```python
from build123d import *

# Parameters (mm, degrees)
F0_W     = 400
F0_H     = 900
F1_DEPTH = 200
F2_SIZE  = 50
F3_R     = 25
F4_R     = 50
F5_DEPTH = 200.001


with BuildPart() as f1:
    # F0 (on Front) → F1 (new body)
    with BuildSketch(Plane.XZ):
        with Locations((0, -35.980602)):
            Rectangle(F0_W, F0_H)
    extrude(amount=F1_DEPTH)

    # F2
    f2_edges = [f1.edges().sort_by_distance(p)[0] for p in [
        (-200, -100, 414.019398),
        (200, -100, 414.019398),
    ]]
    chamfer(f2_edges, length=F2_SIZE)

    # F3
    f3_edges = [f1.edges().sort_by_distance(p)[0] for p in [
        (-200, -100, -485.980602),
        (200, -100, -485.980602),
    ]]
    fillet(f3_edges, radius=F3_R)

    # F4 (on face) → F5 (cut, through all)
    with BuildSketch(Plane.XZ.offset(200)):
        Circle(F4_R)
    extrude(amount=-F5_DEPTH, mode=Mode.SUBTRACT)


solid = f1.part
```
Input: part model. Units: mm. Frame: model coordinates. Coordinates: 2 decimals unless noted, no trailing zeros. Write each loop counter-clockwise with the first axis right and the second up, starting at its lowest first coordinate (ties: lowest second). Pieces come first, ordered by that corner, then holes. Notation, with made-up numbers: M 67,42.5 L 72,42.5 A18 cw 72,58.5 Z; hole C 60.5,77 d7. An arc over 180 degrees is marked long. Use one line per item in the form item = value.
Q1. Section A-A (z = 0). Return loops of the section in (x, y), plus the area to 3 significant figures.
Answer below:
outline = M -200,-200 L -50,-200 L -50,0 L -200,0 Z; M 50,-200 L 200,-200 L 200,0 L 50,0 Z
area = 60,000 mm²
Q2. Section B-B (x = 0). Return loops of the section in (y, z).
Answer below:
outline = M -200,-485.98 L 0,-485.98 L 0,-50 L -200,-50 Z; M -200,50 L 0,50 L 0,414.02 L -200,414.02 Z
Q3. Material intervals for probe 1 along Z at (x, y) = (0, -64); probe 2 along Z at (x, y) = (13, -135); probe 3 along X at (y, z) = (-44.5, -9), sorted ascending. Write a range as from..to.
Answer below:
probe_1 = -485.98..-50, 50..414.02
probe_2 = -485.98..-48.28, 48.28..414.02
probe_3 = -200..-49.18, 49.18..200
Q4. Section C-C (y = -76.5). Return loops of the section in (x, z).
Answer below:
outline = M -200,-460.98 A25 ccw -175,-485.98 L 175,-485.98 A25 ccw 200,-460.98 L 200,364.02 L 150,414.02 L -150,414.02 L -200,364.02 Z; hole C 0,0 d100
Q5. Draft query along X for faces 1 (the face through (-47, 0, -30)), 2 (the face through (-192.871, -101.4, -478.463)), 3 (the face through (200, -99, -54)), 4 (the face through (47.69, -101.4, 15.02)). Return one class per face: released by +X, released by -X, zero draft, split by the parting line, or undercut.
Answer below:
face_1 = zero draft
face_2 = released by -X
face_3 = released by +X
face_4 = undercut
